Model file for the job. Use its own axes, mm. A direction names the side the tool comes from. Coordinates: 2 decimals unless noted, no trailing zeros. Order: outer loops, then holes, each group sorted by start corner. A loop starts at its lowest first (then second) coordinate and runs counter-clockwise, first axis right, second up. Notation, with made-up numbers: M 64,51.5 L 97,51.5 A21 cw 97,65.5 Z; hole C 10.5,-16 d10. An arc over 180 degrees is marked long. Return JSON: item names as keys, results as strings.
```python
from build123d import *

# Parameters (mm, degrees)
BOSS_EXTRUDE1_DEPTH = 35
SHELL1_T            = -2
SKETCH3_R           = 5
BOSS_EXTRUDE2_DEPTH = 35
SKETCH4_R           = 6.188496774
BOSS_EXTRUDE3_DEPTH = 25


with BuildPart() as part:
    # Sketch2 → Boss-Extrude1 (new body)
    with BuildSketch(Plane.XY):
        with BuildLine():
            Line((0, 0), (-44.5203539, 22.758253198))
            ThreePointArc((-44.5203539, 22.758253198), (0, 50), (44.5203539, 22.758253198))
            Line((44.5203539, 22.758253198), (0, 0))
        make_face()
    extrude(amount=BOSS_EXTRUDE1_DEPTH)

    # Shell1
    shell1_openings = [part.faces().sort_by_distance(p)[0] for p in [
        (-22.26017695, 11.379126599, 17.5),
        (22.26017695, 11.379126599, 17.5),
    ]]
    offset(amount=SHELL1_T, openings=shell1_openings, kind=Kind.INTERSECTION)

    # Sketch3 → Boss-Extrude2 (add)
    with BuildSketch(Plane.XY.offset(35)):
        with Locations(Location((0, 0, 0), (0, 0, 27.075555237))):
            Circle(SKETCH3_R)
    extrude(amount=-BOSS_EXTRUDE2_DEPTH)

    # Sketch4 → Boss-Extrude3 (add)
    with BuildSketch(Plane(origin=(0, 49.758126055, 0), x_dir=(1, 0, 0), z_dir=(0, 1, 0))):
        with Locations(Location((0, -17.15723549, 0), (0, 0, 142.53731078))):
            Circle(SKETCH4_R)
    extrude(amount=BOSS_EXTRUDE3_DEPTH)


solid = part.part
```
Item 1: Saw through at A-A (z = 29). Write the cut outline in (x, y).
Check result:
{"outline": "M -44.52,22.76 L -42.74,21.85 A48 cw 42.74,21.85 L 44.52,22.76 A50 ccw Z; C 0,0 d10"}
Item 2: Saw through at B-B (y = 11.5). Write the cut outline in (x, z), and give its area (3 significant figures).
Check result:
{"outline": "M -22.5,0 L 22.5,0 L 22.5,2 L -22.5,2 Z; M -22.5,33 L 22.5,33 L 22.5,35 L -22.5,35 Z", "area": "180 mm2"}
Item 3: 3-axis set-ups, long thin cutter, end or side, ignore diameter. For faces 1 (the cylindrical face through (1.26, -4.84, 17.74)), 2 (the flat face through (-2, 25, 0)), 3 (the cylindrical face through (1.07, 62.08, 11.06)): which of +Z, -Z, +X, -X, +Y, -Y reach the whole face in a straight line?
Check result:
{"face 1": "none", "face 2": "-Z, +X, -X, +Y, -Y", "face 3": "+Y"}
Item 4: Saw through at D-D (y = 45). Write the cut outline in (x, z), and give its area (3 significant figures).
Check result:
{"outline": "M -21.79,0 L 21.79,0 L 21.79,35 L -21.79,35 Z; hole M -16.7,2 L 16.7,2 L 16.7,33 L -16.7,33 Z", "area": "490 mm2"}
Item 5: Saw through at C-C (x = 0). Write the cut outline in (y, z).
Check result:
{"outline": "M -5,0 L 50,0 L 50,10.97 L 74.76,10.97 L 74.76,23.35 L 50,23.35 L 50,35 L -5,35 Z; hole M 5,2 L 48,2 L 48,33 L 5,33 Z"}
Item 6: Pull direction Z, two halves, no side cores. Call faces 4 (the flat face through (1, 25, 2)), 5 (the flat face through (1, 29, 35)), 6 (the flat face through (0, 74.758, 17)): +Z half, -Z half, draft (parallel to the pull), parting line (faces both ways), or undercut.
Check result:
{"face 4": "undercut", "face 5": "+Z half", "face 6": "draft"}
Item 7: Wall check: line 1 (Z direction, x = -18, y = 26.5); line 2 (X direction, y = 63.5, z = 13.5); line 3 (X direction, y = 25, z = 28). Give the ranges that are in metal, low to high.
Check result:
{"line 1": "z = 0 to 2, 33 to 35", "line 2": "x = -4.99 to 4.99", "line 3": "x = -43.3 to -40.98, 40.98 to 43.3"}
Item 8: Drop flat-ended pins along their axis: pin 1 Ø8 at (x, y) = (1.5, 18) entering from -Z; pin 2 Ø12 at (y, z) = (46, 24.5) entering from +X; pin 3 Ø12 at (y, z) = (10, 20) entering from +X. Give the stop position or say it passes through.
Check result:
{"pin 1": "stops at z = 0", "pin 2": "stops at x = 30", "pin 3": "stops at x = 3"}
